Build history of the part. All positions in model axes, mm. Face numbers are marked on the shaded views. A direction names the side the tool comes from. Round coordinates to 2 decimals unless told otherwise and drop trailing zeros. Order: outer loops, then holes, each group sorted by start corner. A loop starts at its lowest first (then second) coordinate and runs counter-clockwise, first axis right, second up. Notation, with made-up numbers: (-7.5, 4.25) -> (42.5, 4.25) arc R25 ccw to (42.5, 16.25) -> close; hole circle Ø11 at (-24, 0). An arc over 180 degrees is marked (long way). Write item = value, one per line.
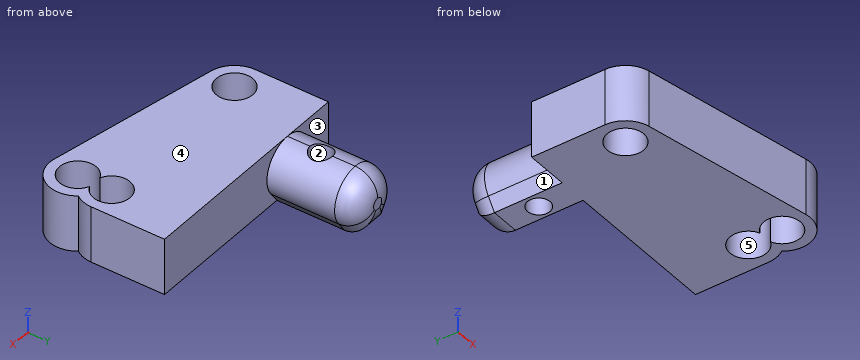
from build123d import *

# Parameters (mm, degrees)
F0_R     = 1.625
F1_DEPTH = 5
F3_DEPTH = 8
F5_R     = 2
F6_R     = 1
F7_DEPTH = 5.001


with BuildPart() as f1:
    # F0 (on Top) → F1 (new body)
    with BuildSketch(Plane.XY):
        with BuildLine():
            Line((-10, 6.5), (-10, 0))
            ThreePointArc((-10, 0), (-9.433355, -1.584972), (-7.99029, -2.451452))
            Line((-7.99029, -2.451452), (7.00971, -5.451452))
            ThreePointArc((7.00971, -5.451452), (9.615017, -4.33293), (9.5, -1.5))
            ThreePointArc((9.5, -1.5), (9.871708, -0.790569), (10, 0))
            Line((10, 0), (10, 6.5))
            Line((10, 6.5), (-10, 6.5))
        make_face()
        with Locations((-7.5, 0)):
            Circle(F0_R, mode=Mode.SUBTRACT)
        with BuildLine():
            ThreePointArc((6.875, -1.5), (7.5, 1.625), (8.125, -1.5))
            ThreePointArc((8.125, -1.5), (7.5, -4.625), (6.875, -1.5))
        make_face(mode=Mode.SUBTRACT)
    extrude(amount=F1_DEPTH)

    # F2 (on face) → F3 (join)
    with BuildSketch(Plane(origin=(0, 6.5, 0), x_dir=(-1, 0, 0), z_dir=(0, 1, 0))):
        with BuildLine():
            Line((6.276674, 0), (7.025208, 1.034212))
            ThreePointArc((7.025208, 1.034212), (7.226485, 3.636998), (5, 5))
            ThreePointArc((5, 5), (2.773515, 3.636998), (2.974792, 1.034212))
            Line((2.974792, 1.034212), (3.723326, 0))
            Line((3.723326, 0), (6.276674, 0))
        make_face()
    extrude(amount=F3_DEPTH)

    # F5
    f5_edges = [f1.edges().sort_by_distance(p)[0] for p in [
        (-3.349059, 14.5, 0.517106),
        (-5, 14.5, 0),
        (-6.650941, 14.5, 0.517106),
        (-5, 14.5, 5),
    ]]
    fillet(f5_edges, radius=F5_R)

    # F6 (on face) → F7 (cut, through all)
    with BuildSketch(Plane(origin=(0, 0, 0), x_dir=(1, 0, 0), z_dir=(0, 0, -1))):
        with Locations((-5, -9.5)):
            Circle(F6_R)
    extrude(amount=-F7_DEPTH, mode=Mode.SUBTRACT)


solid = f1.part
Q1. Cut at A-A, the plane x = 7.5. List the corners of the cut face in (y, z) (3 decimals), and give its area (4 significant figures).
Check values:
outline = (-5.5, 0) -> (-4.625, 0) -> (-4.625, 5) -> (-5.5, 5) -> close; (1.625, 0) -> (6.5, 0) -> (6.5, 5) -> (1.625, 5) -> close
area = 28.75 mm²
Q2. Probe probe 1 along X at (y, z) = (-0.75, 1.9); probe 2 along X at (y, z) = (9.5, 4.3); probe 3 along Y at (x, z) = (-5, 2.8). List the from-to ranges inside material, lowest first.
Check values:
probe_1 = -9.88 to -8.94, -6.06 to 6.06, 8.94 to 9.88
probe_2 = -6.73 to -6, -4 to -3.27
probe_3 = -3.05 to 8.5, 10.5 to 14.5
Q3. Cut at C-C, the plane y = -0.5. List the corners of the cut face in (x, z), and give its area (3 significant figures).
Check values:
outline = (-9.95, 0) -> (-9.05, 0) -> (-9.05, 5) -> (-9.95, 5) -> close; (-5.95, 0) -> (5.95, 0) -> (5.95, 5) -> (-5.95, 5) -> close; (9.05, 0) -> (9.95, 0) -> (9.95, 5) -> (9.05, 5) -> close
area = 68.6 mm²
Q4. Mould opens along Y. For the marked faces 3, 4 and 5 say: released by +Y, released by -Y, zero draft, split by the parting line, or undercut.
Check values:
face_3 = released by +Y
face_4 = zero draft
face_5 = undercut
Q5. Cut at B-B, the plane y = -3. List the corners of the cut face in (x, z) (3 decimals), and give its area (3 significant figures).
Check values:
outline = (-5.248, 0) -> (5.875, 0) -> (5.875, 5) -> (-5.248, 5) -> close; (9.125, 0) -> (10, 0) -> (10, 5) -> (9.125, 5) -> close
area = 60.0 mm²
Q6. Flat gauge pins, fed straight in: pin 1 (2.5 mm diameter, centred on x = 7.5, y = -3, fed in from +Z); pin 2 (1 mm diameter, centred on y = 9.5, z = 0.5, fed in from +X). Where does each tip first touch, or does it go through?
Check values:
pin_1 = through
pin_2 = -3
Q7. Which spindle directions (+Z, -Z, +X, -X, +Y, -Y) get a long thin tool onto all of the face, cutting with end or side? Do the marked faces 1 and 2. Say none if no direction does.
Check values:
face_1 = -Z, -X, +Y
face_2 = +Z, -Z
Q8. Cut at D-D, the plane y = 7.25. List the corners of the cut face in (x, z).
Check values:
outline = (-7.03, 1.03) -> (-6.28, 0) -> (-3.72, 0) -> (-2.97, 1.03) arc R2.5 ccw (long way) to start
